Geometry check sheet. Reference: the model listing, model coordinates, mm. A direction names the side the tool comes from. Give positions to 0.01 mm unless a question says otherwise; leave off trailing zeros. Answer as a JSON object with one key per item and string values.
from build123d import *

# Parameters (mm, degrees)
CHAMFER1_SIZE       = 0.5
BOSS_EXTRUDE1_START = 7
SKETCH2_R           = 53.425
BOSS_EXTRUDE1_DEPTH = 7


with BuildPart() as part:
    # Sketch1 → Revolve1 (revolve)
    with BuildSketch(Plane(origin=(0, 0, 0), x_dir=(1, 0, 0), z_dir=(0, 1, 0)), mode=Mode.PRIVATE) as revolve1_sk:
        Polygon((50.425, 19), (50.425, 14), (48, 14), (48, 0), (51, 0), (51, 2.5), (50, 2.5), (50, 7.5), (51, 7.5), (51, 10), (55, 10), (55, 12), (53.425, 12), (53.425, 19), align=None)
    revolve(revolve1_sk.sketch.rotate(Axis((0, 0, -69.169847328), (0, 0, 1)), 180), axis=Axis((0, 0, -69.169847328), (0, 0, 1)))

    # Chamfer1
    chamfer1_edges = [part.edges().sort_by_distance(p)[0] for p in [
        (51, 0, -10),
        (51, 0, -7.5),
        (50, 0, -7.5),
        (50, 0, -2.5),
        (51, 0, -2.5),
        (51, 0, 0),
        (50.425, 0, -19),
        (53.425, 0, -19),
    ]]
    chamfer(chamfer1_edges, length=CHAMFER1_SIZE - 0.0001)  # a hair under: the kernel refuses the full size

    # Sketch2 → Boss-Extrude1 (add)
    with BuildSketch(Plane(origin=(0, 0, -12), x_dir=(-1, 0, 0), z_dir=(0, 0, -1)).offset(BOSS_EXTRUDE1_START)):
        Circle(SKETCH2_R)
    extrude(amount=-BOSS_EXTRUDE1_DEPTH)


solid = part.part
1) Material ranges on line 1 along Y through (x, z) = (0, -8.25); line 2 along Y through (x, z) = (0, -5.5); line 3 along Z through (x, y) = (-46, 5), recorded low to high. Write a range as from..to.
Geometry check:
{"line 1": "y = -51..-48, 48..51", "line 2": "y = -50..-48, 48..50", "line 3": "z = -19..-12"}
2) Depth check by flat-ended pin: P1, Ø10, axis at y = -39, z = -3.5, coming from the +X side; P2, Ø3, axis at x = 21.5, y = -40.5, coming from the +Z side; P3, Ø2, axis at x = 30.5, z = -15.5, coming from the -Y side. Enter the tip coordinate at first touch or a pass-through.
Geometry check:
{"P1": "stops at x = 37.81", "P2": "stops at z = -12", "P3": "stops at y = -44.54"}
3) Draft check along Z on faces 1 (the face through (45, 18, 0)), 2 (the face through (-25.379, 48.794, -11.014)), 3 (the face through (-47.69, -15.02, -5.03)), 4 (the face through (1, 1, -19)). Enter one of: pulls with the +Z half, pulls with the -Z half, needs draft (parallel to the pull), parting line crosses it, or undercut.
Geometry check:
{"face 1": "pulls with the +Z half", "face 2": "needs draft", "face 3": "undercut", "face 4": "pulls with the -Z half"}
4) Tool access check on faces 5 (the face through (42.396, -32.508, -15.549)), 6 (the face through (-45.783, -14.418, -5.916)). Record the directions out of +Z, -Z, +X, -X, +Y, -Y that give a thin tool (end or side, any length) a straight path to the whole face; none if there is none.
Geometry check:
{"face 5": "-Z", "face 6": "+Z"}
